Autodesk Inventor part; units mm, degrees
ref_plane "작업 평면1" through (0, 21.2, 0) normal (0, 1, 0) x (-1, 0, 0)
ref_plane "YZ Plane" through (0, 0, 0) normal (1, 0, 0) x (0, 1, 0)
ref_plane "XZ Plane" through (0, 0, 0) normal (0, 1, 0) x (-1, 0, 0)
sketch "스케치1" plane through (0, 0, 0) normal (0, 0, 1) x (1, 0, 0)
  circle A0 centre (0, 0) radius 21.2
  dimension "d0" = 42.4
extrude "돌출1" add sketch "스케치1" along normal blind 30
sketch "스케치2" plane through (0, 0, 30) normal (0, 0, 1) x (1, 0, 0)
  circle A0 centre (0, 0) radius 21.2
  dimension "d3" = 42.4
extrude "돌출2" add sketch "스케치2" along normal blind 30
sketch "스케치3" plane through (0, 0, 60) normal (0, 0, 1) x (1, 0, 0)
  circle A0 centre (0, 0) radius 21.2
  dimension "d6" = 42.4
extrude "돌출3" add sketch "스케치3" along normal blind 6
fillet "모깎기1" radius 3 1 edges at (-21.2, 0, 66)
shell "쉘1" thickness 1 removed faces 1 at (2.7392, 4.6861, 0)
ref_plane "작업 평면1" through (0, 21.2, 0) normal (0, 1, 0) x (-1, 0, 0)
sketch "스케치12" plane through (0, 21.2, 0) normal (0, 1, 0) x (-1, 0, 0)
  line L0 (0, 0) -> (0, 60)
  line L1 (0, 60) -> (0, 30)
  line L2 (0, 30) -> (0, 15)
  line L3 (-6, 15) -> (6, 15) construction
  line L4 (-6, 12.5) -> (6, 12.5)
  line L5 (6, 17.5) -> (-6, 17.5)
  arc A0 (-6, 17.5) -> (-6, 12.5) centre (-6, 15) ccw
  arc A1 (6, 12.5) -> (6, 17.5) centre (6, 15) ccw
  dimension "d47" = 60
  dimension "d48" = 30
  dimension "d49" = 15
  dimension "d50" = 6
  dimension "d51" = 5
extrude "돌출12" cut sketch "스케치12" against normal through all
pattern_circular "원형 패턴2" count 4 over 360 about axis through (0, 0, 0) along (0, 0, 1) of "돌출12"
sketch "스케치13" plane through (0, 0, 0) normal (0, 0, -1) x (-1, 0, 0)
  line L0 (0, 0) -> (0, -4)
  line L1 (0, -4) -> (0, 4)
  line L2 (0, 4) -> (20.8192, 4)
  circle A0 centre (0, 0) radius 21.2
  line L3 (0, -4) -> (20.8192, -4)
  dimension "d61" = 4
  dimension "d62" = 8
extrude "돌출13" cut sketch "스케치13" against normal blind 5 contours L1 L2 A0 L3 L0 picked at (6.9397, -2.6667)
properties part number "motor"
Could you check a few things on this model? Use its own coordinates, in mm. A direction names the side the tool comes from. Round coordinates to 2 decimals unless told otherwise and drop trailing zeros. Write each loop counter-clockwise with the first axis right and the second up, starting at its lowest first coordinate (ties: lowest second). Pieces come first, ordered by that corner, then holes. Notation, with made-up numbers: (11.25, -2.5) - (61.25, -2.5) arc R22 ccw to (61.25, 28.5) - close; hole circle Ø8 at (-33.5, -7). An arc over 180 degrees is marked (long way). Put each result on its own line as item: value. Start each with the question number.
(1) Will these pins go through, and if not, where does the flat tip stop? pin 1 (10 mm diameter, centred on y = 12, z = 42, fed in from -X); pin 2 (6 mm diameter, centred on x = -14.5, z = 10, fed in from +Y); pin 3 (2 mm diameter, centred on x = -20.5, y = 0.5, fed in from +Z).
(2) I want a section at C-C, the plane z = 29. Please give me the cut outline in (x, y), plus the area to 3 significant figures.
(3) Thinking about a two-plate mould opening in X: for faces 4 (the flat face through (19, -8, 0)), 5 (the cylindrical face through (-8.5, -19.1, 14.9)), 6 (the cylindrical face through (19.583, 8.12, 31.059)), which applies, released by +X, released by -X, zero draft, split by the parting line, or undercut?
(4) I want a section at B-B, the plane z = 15. Please give me the cut outline in (x, y), plus the area to 3 significant figures.
(5) I need wall thicknesses on probe 1 along X at (y, z) = (0, 27); probe 2 along Y at (x, z) = (-6, 42.5). Which ranges of each line are inside material? Lowest first, please.
(6) I want a section at A-A, the plane x = 0. Please give me the cut outline in (y, z), plus the area to 3 significant figures.
(7) For faces 1 (the flat face through (0, 0, 65)), 2 (the flat face through (0.1, 20.5, 12.5)), 3 (the flat face through (20.4, -0.1, 17.5)), which set-ups out of +Z, -Z, +X, -X, +Y, -Y let a thin tool reach every point of the face, with its end or its side?
Here are the results:
1. pin 1: stops at x = -20.01
1. pin 2: stops at y = 17.81
1. pin 3: stops at z = 65.7
2. outline: circle Ø42.4 at (0, 0); hole circle Ø40.4 at (0, 0)
2. area: 130 mm^2
3. face 4: zero draft
3. face 5: undercut
3. face 6: split by the parting line
4. outline: (-19.42, -8.5) arc R21.2 ccw to (-8.5, -19.42) - (-8.5, -18.32) arc R20.2 cw to (-18.32, -8.5) - close; (-19.42, 8.5) - (-18.32, 8.5) arc R20.2 cw to (-8.5, 18.32) - (-8.5, 19.42) arc R21.2 ccw to start; (8.5, -19.42) arc R21.2 ccw to (19.42, -8.5) - (18.32, -8.5) arc R20.2 cw to (8.5, -18.32) - close; (8.5, 18.32) arc R20.2 cw to (18.32, 8.5) - (19.42, 8.5) arc R21.2 ccw to (8.5, 19.42) - close
4. area: 60.0 mm^2
5. probe 1: x = -21.2 to -20.2, 20.2 to 21.2
5. probe 2: y = -20.33 to -19.29, 19.29 to 20.33
6. outline: (-21.2, 0) - (-20.2, 0) - (-20.2, 12.5) - (-21.2, 12.5) - close; (-21.2, 17.5) - (-20.2, 17.5) - (-20.2, 63) arc R2 cw to (-18.2, 65) - (18.2, 65) arc R2 cw to (20.2, 63) - (20.2, 17.5) - (21.2, 17.5) - (21.2, 63) arc R3 ccw to (18.2, 66) - (-18.2, 66) arc R3 ccw to (-21.2, 63) - close; (20.2, 0) - (21.2, 0) - (21.2, 12.5) - (20.2, 12.5) - close
6. area: 160 mm^2
7. face 1: -Z
7. face 2: +Y, -Y
7. face 3: +X, -X
